Autodesk Inventor part; units mm, degrees
ref_plane "YZ Plane" through (0, 0, 0) normal (1, 0, 0) x (0, 1, 0)
ref_plane "XZ Plane" through (0, 0, 0) normal (0, 1, 0) x (-1, 0, 0)
ref_plane "XY Plane" through (0, 0, 0) normal (0, 0, 1) x (1, 0, 0)
sketch "Skizze1" plane through (0, 0, 0) normal (1, 0, 0) x (0, 1, 0)
  line L0 (0, 0) -> (158, 0)
  line L1 (158, 0) -> (158, -20)
  line L2 (158, -20) -> (0, -20)
  line L3 (0, -20) -> (0, 0)
  dimension "d0" = 158
  dimension "d1" = 20
extrude "Extrusion1" add sketch "Skizze1" along normal blind 10
sketch "Skizze2" plane through (10, 0, 0) normal (1, 0, 0) x (0, 0, -1)
  line L0 (0, 0) -> (20, 0)
  line L1 (20, 0) -> (20, 158)
  point P0 (10, 150)
  dimension "d11" = 150
  dimension "d12" = 10
hole "Bohrung1" at (10, 150, -10) direction (-1, 0, 0) diameter 10.2 end through all
fillet "Rundung1" radius 10 2 edges at (5, 158, 0) (5, 158, -20)
properties part number "HolzHalter"
CAD build for the part. Positions are in the model's coordinates, mm. Coordinates: 2 decimals unless noted, no trailing zeros. Write each loop counter-clockwise with the first axis right and the second up, starting at its lowest first coordinate (ties: lowest second). Pieces come first, ordered by that corner, then holes. Notation, with made-up numbers: (87.25, -11) - (115.25, -11) arc R13 cw to (115.25, 13) - close; hole circle Ø8 at (30, 51). An arc over 180 degrees is marked (long way). Use a Markdown table: item, result. Add a question column.
Item 1: Band-saw the part on C-C, the plane z = -2.5. Give the cut face in (x, y), and give its area (3 significant figures).
Item 2: Band-saw the part on B-B, the plane y = 150. Give the cut face in (x, z), and give its area (3 significant figures).
Item 3: Mould opens along Z. For faces 1 (the face through (5.07, 154.99, -17.15)), 2 (the face through (5, 73, 0)), 3 (the face through (0, 78, -10)), 4 (the face through (5, 155, -9)) say: pulls with the +Z half, pulls with the -Z half, needs draft (parallel to the pull), parting line crosses it, or undercut.
Item 4: Drill centre lines: L1, parallel to Y at x = 4, z = -10; L2, parallel to Y at x = 6.25, z = -13; L3, parallel to Z at x = 5, y = 150. Where is each one in solid material? Low to high. Write a range as from..to.
Item 5: Flat gauge pins, fed straight in: pin 1 (1.5 mm diameter, centred on x = 5.5, z = -3.5, fed in from +Y); pin 2 (1 mm diameter, centred on x = 5, y = 132, fed in from +Z); pin 3 (3 mm diameter, centred on x = 3.5, z = -5, fed in from +Y). Where does each tip first touch, or does it go through?
Numbers:
| question | item | result |
|---|---|---|
| 1 | outline | (0, 0) - (10, 0) - (10, 154.61) - (0, 154.61) - close |
| 1 | area | 1,550 mm2 |
| 2 | outline | (0, -19.8) - (10, -19.8) - (10, -15.1) - (0, -15.1) - close; (0, -4.9) - (10, -4.9) - (10, -0.2) - (0, -0.2) - close |
| 2 | area | 94.0 mm2 |
| 3 | face 1 | pulls with the -Z half |
| 3 | face 2 | pulls with the +Z half |
| 3 | face 3 | needs draft |
| 3 | face 4 | undercut |
| 4 | L1 | 0..144.9, 155.1..158 |
| 4 | L2 | 0..145.88, 154.12..157.54 |
| 4 | L3 | -19.8..-15.1, -4.9..-0.2 |
| 5 | pin 1 | y = 156.18 |
| 5 | pin 2 | z = 0 |
| 5 | pin 3 | y = 157.37 |
